CAD build for the part. Positions are in the model's coordinates, mm. A direction names the side the tool comes from. Give positions to 0.01 mm unless a question says otherwise; leave off trailing zeros. Loops run counter-clockwise (first coordinate to the right, second up) from the corner with the lowest first, then second, coordinate; pieces in that order, holes last. Notation, with made-up numbers: (38.25, 41) -> (67.25, 41) arc R26 ccw to (67.25, 78) -> close; hole circle Ø9 at (-21, 39). An arc over 180 degrees is marked (long way). Use one line per item in the form item = value.
```python
from build123d import *

# Parameters (mm, degrees)
F1_DEPTH = 16
F3_D     = 4
F3_DEPTH = 30
F3_TIP   = 1.2017212381
F4_R     = 1
F5_R     = 7.99999
F6_DEPTH = 2.54


# Not quite as in the source:
# - a fillet or chamfer is up to 0.001 mm smaller than in the source, because OpenCascade refuses the exact size


with BuildPart() as f1:
    # F0 (on Top) → F1 (new body)
    with BuildSketch(Plane.XY):
        Polygon((0, 23), (0, 18), (22.5, 18), (22.5, 0), (0, 0), (0, -5), (27.5, -5), (27.5, 23), align=None)
    extrude(amount=F1_DEPTH)

    # F3
    with Locations(Plane.XZ.offset(5)):
        with Locations((8, 8)):
            Hole(F3_D / 2, depth=F3_DEPTH)
            with Locations((0, 0, -(F3_DEPTH + F3_TIP / 2))):  # 118° drill point
                Cone(0, F3_D / 2, F3_TIP, mode=Mode.SUBTRACT)

    # F4
    f4_edges = [f1.edges().sort_by_distance(p)[0] for p in [
        (22.5, 18, 8),
        (22.5, 0, 8),
        (27.5, -5, 8),
        (27.5, 23, 8),
    ]]
    fillet(f4_edges, radius=F4_R)

    # F5 (radius 8 in the source; OpenCascade refuses exactly that, so slightly less here)
    f5_edges = [f1.edges().sort_by_distance(p)[0] for p in [
        (0, -2.5, 16),
        (0, 20.5, 16),
        (0, -2.5, 0),
        (0, 20.5, 0),
    ]]
    fillet(f5_edges, radius=F5_R)

    # F2 (on face) → F6 (cut)
    with BuildSketch(Plane.XZ.offset(5)):
        Polygon((11, 6.2679491924), (11, 9.7320508076), (8, 11.4641016151), (5, 9.7320508076), (5, 6.2679491924), (8, 4.5358983849), align=None)
    extrude(amount=-F6_DEPTH, mode=Mode.SUBTRACT)


solid = f1.part
```
1. Drop flat-ended pins along their axis: P1, Ø2.5, axis at x = 8, z = 8, coming from the +Y side; P2, Ø1.3, axis at y = -3.5, z = 9, coming from the -X side; P3, Ø4, axis at y = 5, z = 3, coming from the -X side. Give the stop position or say it passes through.
Result sheet:
P1 = through
P2 = 0.01
P3 = 22.5
2. Tool access for faces 1 (the cylindrical face through (22.199, 17.715, 8.112)), 2 (the flat face through (24, 9, 16)), 3 (the flat face through (6.5, -3.7, 10.6)): list every direction of +Z, -Z, +X, -X, +Y, -Y with a clear straight run to the whole face (end or side of a thin tool).
Result sheet:
face_1 = +Z, -Z, -X
face_2 = +Z, +X, -X, +Y, -Y
face_3 = -Y
3. Mould opens along Y. For faces 4 (the flat face through (11, 18, 8)), 5 (the flat face through (13, -5, 8)), 6 (the flat face through (9.5, -3.7, 5.4)) say: pulls with the +Y half, pulls with the -Y half, needs draft (parallel to the pull), parting line crosses it, or undercut.
Result sheet:
face_4 = undercut
face_5 = pulls with the -Y half
face_6 = needs draft
4. Cut at A-A, the plane x = 16.25. Write the cut outline in (y, z).
Result sheet:
outline = (-5, 0) -> (0, 0) -> (0, 16) -> (-5, 16) -> close; (18, 0) -> (23, 0) -> (23, 16) -> (18, 16) -> close
5. Cut at D-D, the plane x = 2.75. Write the cut outline in (y, z).
Result sheet:
outline = (-5, 1.96) -> (0, 1.96) -> (0, 14.04) -> (-5, 14.04) -> close; (18, 1.96) -> (23, 1.96) -> (23, 14.04) -> (18, 14.04) -> close
6. Drill centre lines: line 1 (Y direction, x = 20.25, z = 2.25); line 2 (Z direction, x = 8, y = 21.15); line 3 (X direction, y = 2.5, z = 11.75). Where is each one in solid material? Low to high.
Result sheet:
line_1 = -5 to 0, 18 to 23
line_2 = 0 to 6, 10 to 16
line_3 = 22.5 to 27.5
7. Cut at C-C, the plane z = 12.25. Write the cut outline in (x, y).
Result sheet:
outline = (1.22, -5) -> (26.5, -5) arc R1 ccw to (27.5, -4) -> (27.5, 22) arc R1 ccw to (26.5, 23) -> (1.22, 23) -> (1.22, 18) -> (21.5, 18) arc R1 cw to (22.5, 17) -> (22.5, 1) arc R1 cw to (21.5, 0) -> (1.22, 0) -> close
